Read the model definition and answer for the solid it produces. Units are mm, in the model's axes. Give positions to 0.01 mm unless a question says otherwise; leave off trailing zeros. Order: outer loops, then holes, each group sorted by start corner. A loop starts at its lowest first (then second) coordinate and runs counter-clockwise, first axis right, second up.
```python
from build123d import *

# Parameters (mm, degrees)
F1_DEPTH = 1
F2_D     = 0.5
F2_DEPTH = 17
F2_TIP   = 0.1502151548


with BuildPart() as f1:
    # F0 (on Top) → F1 (new body)
    with BuildSketch(Plane.XY):
        with BuildLine():
            add(Edge.make_bspline(
                [(-6.8700691129, 10.142221176), (-8.399545307, 9.5712927005), (-10.6213726103, 7.7990288846), (-9.4482654422, 10.3310348046)],
                knots=[0.5589666429, 0.5589666429, 0.5589666429, 0.5589666429, 1, 1, 1, 1], degree=3))
            add(Edge.make_bspline(
                [(-2.7175999736, 10.142221176), (-4.1052754968, 9.659698233), (-4.9316076337, 10.8658171767), (-6.8700691129, 10.142221176)],
                knots=[0, 0, 0, 0, 0.5589666429, 0.5589666429, 0.5589666429, 0.5589666429], degree=3))
            Line((-2.7175999736, 10.142221176), (-3.6234666314, 13.522961568))
            ThreePointArc((-3.6234666314, 13.522961568), (-6.727900413, 12.2774327949), (-9.4482654422, 10.3310348046))
        make_face()
        with BuildLine():
            ThreePointArc((6.8700691129, 10.142221176), (0, -12.25), (-6.8700691129, 10.142221176))
            add(Edge.make_bspline(
                [(-6.8700691129, 10.142221176), (-8.399545307, 9.5712927005), (-10.6213726103, 7.7990288846), (-9.4482654422, 10.3310348046)],
                knots=[0.5589666429, 0.5589666429, 0.5589666429, 0.5589666429, 1, 1, 1, 1], degree=3))
            ThreePointArc((-9.4482654422, 10.3310348046), (0, -14), (9.4482654422, 10.3310348046))
            add(Edge.make_bspline(
                [(6.8700691129, 10.142221176), (8.3520722793, 9.6407168218), (10.2458875626, 8.1284232438), (9.4482654422, 10.3310348046)],
                knots=[0.5589666429, 0.5589666429, 0.5589666429, 0.5589666429, 1, 1, 1, 1], degree=3))
        make_face()
        with BuildLine():
            add(Edge.make_bspline(
                [(2.7175999736, 10.142221176), (3.7749782205, 9.7897974774), (4.9917750531, 10.7778288933), (6.8700691129, 10.142221176)],
                knots=[0, 0, 0, 0, 0.5589666429, 0.5589666429, 0.5589666429, 0.5589666429], degree=3))
            add(Edge.make_bspline(
                [(6.8700691129, 10.142221176), (8.3520722793, 9.6407168218), (10.2458875626, 8.1284232438), (9.4482654422, 10.3310348046)],
                knots=[0.5589666429, 0.5589666429, 0.5589666429, 0.5589666429, 1, 1, 1, 1], degree=3))
            ThreePointArc((9.4482654422, 10.3310348046), (6.727900413, 12.2774327949), (3.6234666314, 13.522961568))
            Line((3.6234666314, 13.522961568), (2.7175999736, 10.142221176))
        make_face()
        with BuildLine():
            Line((-3.6234666314, 13.522961568), (-2.7175999736, 10.142221176))
            ThreePointArc((-2.7175999736, 10.142221176), (-1.4801631065, 12.285524701), (-3.6234666314, 13.522961568))
        make_face()
        with BuildLine():
            ThreePointArc((3.6234666314, 13.522961568), (1.4801631065, 12.285524701), (2.7175999736, 10.142221176))
            Line((2.7175999736, 10.142221176), (3.6234666314, 13.522961568))
        make_face()
    extrude(amount=F1_DEPTH)

    # F2
    with Locations(Plane(origin=(0, 0, 0), x_dir=(1, 0, 0), z_dir=(0, 0, -1))):
        with Locations((-3.1705333025, -11.832591372), (3.1705333025, -11.832591372)):
            Hole(F2_D / 2, depth=F2_DEPTH)
            with Locations((0, 0, -(F2_DEPTH + F2_TIP / 2))):  # 118° drill point
                Cone(0, F2_D / 2, F2_TIP, mode=Mode.SUBTRACT)


solid = f1.part
```
1) The part is cut by section A-A on y = -10.75. Determine the outline of the cut face in (x, z).
Final values:
outline: (-8.97, 0) - (-5.87, 0) - (-5.87, 1) - (-8.97, 1) - close; (5.87, 0) - (8.97, 0) - (8.97, 1) - (5.87, 1) - close
2) For a pull along X with two mould halves and no side action, classify faces 1 (the face through (-1.47, 12.25, 0.49)), 2 (the face through (2, 11, 1)) as released by +X, released by -X, zero draft, split by the parting line, or undercut.
Final values:
face 1: undercut
face 2: zero draft
3) The part is cut by section B-B on y = 0. Determine the outline of the cut face in (x, z).
Final values:
outline: (-14, 0) - (-12.25, 0) - (-12.25, 1) - (-14, 1) - close; (12.25, 0) - (14, 0) - (14, 1) - (12.25, 1) - close
4) The part is cut by section D-D on z = 0.6. Count the separate pieces of the cut face and the enclosed holes in it, and give its area (3 significant figures).
Final values:
separate pieces: 1
enclosed holes: 2
area: 149 mm2
5) The part is cut by section C-C on x = 0. Determine the outline of the cut face in (y, z).
Final values:
outline: (-14, 0) - (-12.25, 0) - (-12.25, 1) - (-14, 1) - close
6) Consider L1, parallel to X at y = 0, z = 0.25; L2, parallel to Y at x = -3, z = 0.9; L3, parallel to Y at x = -2.75, z = 0.1. Determine where each line is inside the solid, lowest interval first.
Final values:
L1: x = -14 to -12.25, 12.25 to 14
L2: y = -13.67 to -11.88, 10.06 to 11.65, 12.02 to 13.57
L3: y = -13.73 to -11.94, 10.13 to 13.53
